Input: dimensioned drawing with shaded views. Units: mm. Origin: part minimum x, y, z. Coordinates: 2 decimals unless noted, no trailing zeros. Order: outer loops, then holes, each group sorted by start corner. A loop starts at its lowest first (then second) coordinate and runs counter-clockwise, first axis right, second up. Notation, with made-up numbers: (-13.75, 19.25) -> (27.25, 19.25) arc R14 cw to (27.25, 42.25) -> close; hole circle Ø11 at (10, 54.5). An arc over 180 degrees is marked (long way). Answer as CSV lines item,"result".
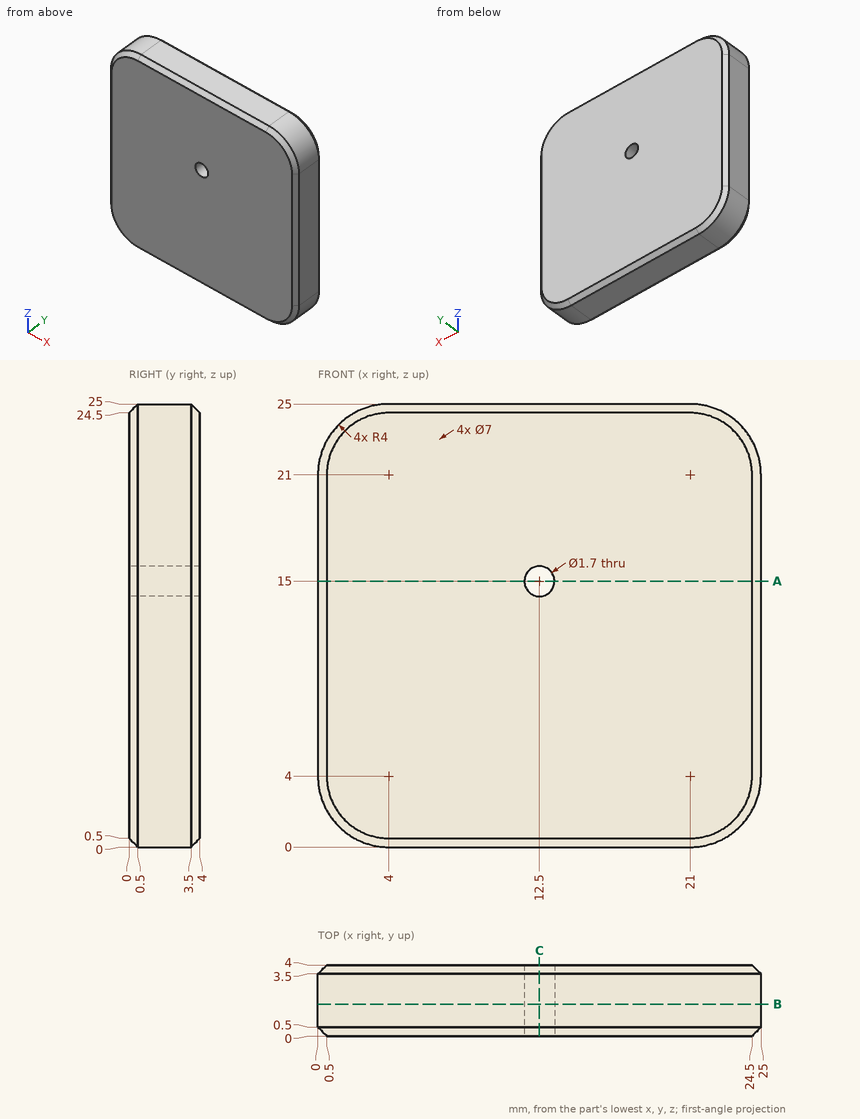
1. Ray query, line 1 along X through (y, z) = (1.3, 15); line 2 along Z through (x, y) = (12, 3.65); line 3 along Z through (x, y) = (22.5, 2.5). Return the intervals inside material, ascending.
Findings:
line 1,"x = 0 to 11.65, 13.35 to 25"
line 2,"z = 0.15 to 14.31, 15.69 to 24.85"
line 3,"z = 0.29 to 24.71"
2. Contact query for a flat-ended pin moving along its axis: pin 1 (2 mm diameter, centred on x = 11, y = 2.5, fed in from -Z). Output: stop coordinate, or through.
Findings:
pin 1,"stops at z = 0"
3. Cut plane C-C (x = 12.5). Return the cut outline in (y, z).
Findings:
outline,"(0, 0.5) -> (0.5, 0) -> (3.5, 0) -> (4, 0.5) -> (4, 14.15) -> (0, 14.15) -> close; (0, 15.85) -> (4, 15.85) -> (4, 24.5) -> (3.5, 25) -> (0.5, 25) -> (0, 24.5) -> close"
4. Cut plane A-A (z = 15). Return the cut outline in (x, y).
Findings:
outline,"(0, 0.5) -> (0.5, 0) -> (11.65, 0) -> (11.65, 4) -> (0.5, 4) -> (0, 3.5) -> close; (13.35, 0) -> (24.5, 0) -> (25, 0.5) -> (25, 3.5) -> (24.5, 4) -> (13.35, 4) -> close"
5. Cut plane B-B (y = 1.8). Return the cut outline in (x, z), plus the area to 3 significant figures.
Findings:
outline,"(0, 4) arc R4 ccw to (4, 0) -> (21, 0) arc R4 ccw to (25, 4) -> (25, 21) arc R4 ccw to (21, 25) -> (4, 25) arc R4 ccw to (0, 21) -> close; hole circle Ø1.7 at (12.5, 15)"
area,"609 mm2"
